Work out the finished part from the listing and answer in its coordinate system (mm). A direction names the side the tool comes from. Coordinates: 2 decimals unless noted, no trailing zeros. Order: outer loops, then holes, each group sorted by start corner. A loop starts at its lowest first (then second) coordinate and runs counter-clockwise, first axis right, second up. Notation, with made-up numbers: M 7.5,-2 L 53.5,-2 A17 ccw 53.5,5 Z; hole C 20.5,78.5 d1. An arc over 180 degrees is marked long. Use a Markdown table: item, result. Add a question column.
from build123d import *

# Parameters (mm, degrees)
BOSS_EXTRUDE1_DEPTH         = 65
BOSS_EXTRUDE1_DEPTH_BACK    = 60
BOSS_EXTRUDE2_DEPTH         = 50
BOSS_EXTRUDE2_DEPTH_BACK    = 50
BOSS_EXTRUDE3_START         = -7
BOSS_EXTRUDE3_DEPTH         = 7
SKETCH6_R                   = 2
CUT_EXTRUDE1_DEPTH          = 5
M3_TAPPED_HOLE1_D           = 2.5
M3_TAPPED_HOLE1_DEPTH       = 7.5
M3_TAPPED_HOLE1_CSINK_D     = 3.05
M3_TAPPED_HOLE1_CSINK_ANGLE = 90
M3_TAPPED_HOLE1_TIP         = 0.751075774


with BuildPart() as part:
    # Sketch1 → Boss-Extrude1 (new, two sides: drawn at the far end of the back side and taken through both)
    with BuildSketch(Plane.XY.offset(-BOSS_EXTRUDE1_DEPTH_BACK)):
        with BuildLine():
            Line((9.013878189, 15), (0, 15))
            Line((0, 15), (0, 10))
            ThreePointArc((0, 10), (7.071067812, 7.071067812), (10, 0))
            ThreePointArc((10, 0), (7.071067812, -7.071067812), (0, -10))
            Line((0, -10), (0, -15))
            Line((0, -15), (9.013878189, -15))
            ThreePointArc((9.013878189, -15), (15.231429157, -8.617050879), (17.5, 0))
            ThreePointArc((17.5, 0), (15.231429157, 8.617050879), (9.013878189, 15))
        make_face()
        with BuildLine():
            Line((0, 10), (0, 15))
            Line((0, 15), (-9.013878189, 15))
            ThreePointArc((-9.013878189, 15), (-17.5, 0), (-9.013878189, -15))
            Line((-9.013878189, -15), (0, -15))
            Line((0, -15), (0, -10))
            ThreePointArc((0, -10), (-10, 0), (0, 10))
        make_face()
    extrude(amount=BOSS_EXTRUDE1_DEPTH + BOSS_EXTRUDE1_DEPTH_BACK)

    # Sketch1_23 → Boss-Extrude2 (add, two sides: drawn at the far end of the back side and taken through both)
    with BuildSketch(Plane.XY.offset(-BOSS_EXTRUDE2_DEPTH_BACK)):
        with BuildLine():
            Line((-9.013878189, 15), (-10.828203914, 15))
            ThreePointArc((-10.828203914, 15), (-18.5, 0), (-10.828203914, -15))
            Line((-10.828203914, -15), (-9.013878189, -15))
            ThreePointArc((-9.013878189, -15), (-17.5, 0), (-9.013878189, 15))
        make_face()
        with BuildLine():
            ThreePointArc((18.5, 0), (16.470758519, 8.42402005), (10.828203914, 15))
            Line((10.828203914, 15), (9.013878189, 15))
            ThreePointArc((9.013878189, 15), (15.231429157, 8.617050879), (17.5, 0))
            ThreePointArc((17.5, 0), (15.231429157, -8.617050879), (9.013878189, -15))
            Line((9.013878189, -15), (10.828203914, -15))
            ThreePointArc((10.828203914, -15), (16.470758519, -8.42402005), (18.5, 0))
        make_face()
    extrude(amount=BOSS_EXTRUDE2_DEPTH + BOSS_EXTRUDE2_DEPTH_BACK)

    # Sketch5 → Boss-Extrude3 (add)
    with BuildSketch(Plane.XY.offset(65).offset(BOSS_EXTRUDE3_START)):
        with BuildLine():
            ThreePointArc((9.013878189, 15), (0, 17.5), (-9.013878189, 15))
            Line((-9.013878189, 15), (9.013878189, 15))
        make_face()
        with BuildLine():
            ThreePointArc((-9.013878189, -15), (0, -17.5), (9.013878189, -15))
            Line((9.013878189, -15), (-9.013878189, -15))
        make_face()
    extrude(amount=BOSS_EXTRUDE3_DEPTH)

    # Sketch6 → Cut-Extrude1 (cut)
    with BuildSketch(Plane.XY.offset(65)):
        with Locations((0, 14.25)):
            Circle(SKETCH6_R)
        with Locations((12.340862004, -7.125)):
            Circle(SKETCH6_R)
        with Locations((-12.340862004, -7.125)):
            Circle(SKETCH6_R)
    extrude(amount=-CUT_EXTRUDE1_DEPTH, mode=Mode.SUBTRACT)

    # M3 Tapped Hole1
    with Locations(Plane(origin=(0, -15, 0), x_dir=(-1, 0, 0), z_dir=(0, -1, 0))):
        with Locations((0, 0)):
            CounterSinkHole(M3_TAPPED_HOLE1_D / 2, M3_TAPPED_HOLE1_CSINK_D / 2, depth=M3_TAPPED_HOLE1_DEPTH, counter_sink_angle=M3_TAPPED_HOLE1_CSINK_ANGLE)
            with Locations((0, 0, -(M3_TAPPED_HOLE1_DEPTH + M3_TAPPED_HOLE1_TIP / 2))):  # 118° drill point
                Cone(0, M3_TAPPED_HOLE1_D / 2, M3_TAPPED_HOLE1_TIP, mode=Mode.SUBTRACT)


solid = part.part
(1) A cutting plane is placed at A-A on z = 0. Write down the section's boundary in (x, y) (3 decimals).
(2) Given P1, Ø1, axis at x = 10.5, z = -42, coming from the -Y side; P2, Ø3, axis at x = -12.5, y = -7, coming from the +Z side; P3, Ø8, axis at y = 6, z = 14.5, coming from the +X side, each flat-ended and moving along its own axis, determine where each tip first touches the part or whether it passes through.
(3) Which of the six approach directions +Z, -Z, +X, -X, +Y, -Y give full straight-line access (tool end or side, diameter ignored) to faces 1 (the cylindrical face through (-0.27, -12.29, 1.22)), 2 (the flat face through (0, -15, -2)), 3 (the cylindrical face through (-0.26, 16.233, 62.535))?
(4) A cutting plane is placed at D-D on x = -13. Write down the section's boundary in (y, z), plus the area to 3 significant figures.
(5) Straight lines are drawn through the part: line 1 (Y direction, x = 0, z = 61.8); line 2 (Y direction, x = 0.5, z = -4.5); line 3 (Y direction, x = 15, z = -35.5). For each, find the intervals that lie inside material, in ascending order.
(6) A cutting plane is placed at B-B on x = -6.5. Write down the section's boundary in (y, z), plus the area to 3 significant figures.
(7) A cutting plane is placed at C-C on y = -11.5. Write down the section's boundary in (x, z).
(8) The mould has two halves that part along Y. Classify faces 4 (the flat face through (-0.2, 10.2, -60)), 5 (the cylindrical face through (-14.34, -7.04, 62.54)), 6 (the flat face through (0, 15, -2)), 7 (the flat face through (0, 14, 60)): pulls with the +Y half, pulls with the -Y half, needs draft (parallel to the pull), parting line crosses it, or undercut.
From the geometry:
| question | item | result |
|---|---|---|
| 1 | outline | M -10.828,-15 L -1.525,-15 L -1.25,-14.725 L -1.25,-9.922 A10 cw long 1.25,-9.922 L 1.25,-14.725 L 1.525,-15 L 10.828,-15 A18.5 ccw 10.828,15 L -10.828,15 A18.5 ccw Z |
| 2 | P1 | stops at y = -15 |
| 2 | P2 | stops at z = 60 |
| 2 | P3 | stops at x = 18.39 |
| 3 | face 1 | -Y |
| 3 | face 2 | -Z, +X, -X, -Y |
| 3 | face 3 | +Z |
| 4 | outline | M -13.16,-50 L -11.72,-50 L -11.72,-60 L 11.72,-60 L 11.72,-50 L 13.16,-50 L 13.16,50 L 11.72,50 L 11.72,65 L -5.24,65 L -5.24,60 L -9.01,60 L -9.01,65 L -11.72,65 L -11.72,50 L -13.16,50 Z |
| 4 | area | 3,200 mm2 |
| 5 | line 1 | y = -17.5 to -10, 10 to 12.25, 16.25 to 17.5 |
| 5 | line 2 | y = -15 to -9.99, 9.99 to 15 |
| 5 | line 3 | y = -10.83 to 10.83 |
| 6 | outline | M -16.25,58 L -15,58 L -15,-60 L -7.6,-60 L -7.6,65 L -16.25,65 Z; M 7.6,-60 L 15,-60 L 15,58 L 16.25,58 L 16.25,65 L 7.6,65 Z |
| 6 | area | 1,870 mm2 |
| 7 | outline | M -14.49,-50 L -13.19,-50 L -13.19,-60 L 13.19,-60 L 13.19,-50 L 14.49,-50 L 14.49,50 L 13.19,50 L 13.19,65 L -13.19,65 L -13.19,50 L -14.49,50 Z; hole C 0,0 d2.5 |
| 8 | face 4 | needs draft |
| 8 | face 5 | undercut |
| 8 | face 6 | pulls with the +Y half |
| 8 | face 7 | undercut |
